Design review of the part built by this model. Coordinates are the model's own, in mm. Face numbers are marked on the shaded views. Round coordinates to 2 decimals unless told otherwise and drop trailing zeros. Use one line per item in the form item = value.
```python
from build123d import *

# Parameters (mm, degrees)
F0_W     = 539.75
F0_H     = 304.8
F0_W_2   = 15.24
F0_H_2   = 58.42
F0_W_3   = 304.8
F0_H_3   = 12.7
F0_R     = 47.625
F0_W_4   = 69.85
F0_H_4   = 7.62
F1_DEPTH = 12.7
F0_W_5   = 10.4902
F0_H_5   = 4.572
F2_DEPTH = 2.54
F0_R_2   = 41.275
F3_DEPTH = 12.7
F4_DEPTH = 5.08
F5_R     = 12.7
F6_R     = 5.08
F7_R     = 2.54
F8_R     = 2.032


with BuildPart() as f1:
    # F0 (on Top) → F1 (new body)
    with BuildSketch(Plane.XY):
        Rectangle(F0_W, F0_H)
        with Locations((-245.098478, -86.36)):
            Rectangle(F0_W_2, F0_H_2, mode=Mode.SUBTRACT)
        with Locations((-66.675, -107.95)):
            Rectangle(F0_W_3, F0_H_3, mode=Mode.SUBTRACT)
        with Locations((-66.675, -70.889322)):
            Rectangle(F0_W_3, F0_H_3, mode=Mode.SUBTRACT)
        with Locations((-66.675, -33.828645)):
            Rectangle(F0_W_3, F0_H_3, mode=Mode.SUBTRACT)
        with Locations((245.098478, -86.36)):
            Rectangle(F0_W_2, F0_H_2, mode=Mode.SUBTRACT)
        with Locations((-66.675, 3.232033)):
            Rectangle(F0_W_3, F0_H_3, mode=Mode.SUBTRACT)
        with Locations((-66.675, 40.292711)):
            Rectangle(F0_W_3, F0_H_3, mode=Mode.SUBTRACT)
        with Locations((-245.098478, 86.36)):
            Rectangle(F0_W_2, F0_H_2, mode=Mode.SUBTRACT)
        with Locations((-66.675, 77.353389)):
            Rectangle(F0_W_3, F0_H_3, mode=Mode.SUBTRACT)
        with Locations((-66.675, 114.414066)):
            Rectangle(F0_W_3, F0_H_3, mode=Mode.SUBTRACT)
        with Locations((177.8, 18.529066)):
            Circle(F0_R, mode=Mode.SUBTRACT)
        with Locations((245.098478, 86.36)):
            Rectangle(F0_W_2, F0_H_2, mode=Mode.SUBTRACT)
        with Locations((177.8, 120.764066)):
            Rectangle(F0_W_4, F0_H_4, mode=Mode.SUBTRACT)
    extrude(amount=F1_DEPTH)

    # F0 (on Top) → F2 (join)
    with BuildSketch(Plane.XY):
        with Locations((177.8, 120.764066)):
            Rectangle(F0_W_4, F0_H_4)
        with Locations((177.8, 120.764066)):
            Rectangle(F0_W_5, F0_H_5, mode=Mode.SUBTRACT)
    extrude(amount=F2_DEPTH)

    # F0 (on Top) → F3 (join)
    with BuildSketch(Plane.XY):
        with Locations((177.8, 18.529066)):
            Circle(F0_R)
        with Locations((177.8, 18.529066)):
            Circle(F0_R_2, mode=Mode.SUBTRACT)
    extrude(amount=F3_DEPTH)

    # F0 (on Top) → F4 (join)
    with BuildSketch(Plane.XY):
        with Locations((177.8, 18.529066)):
            Circle(F0_R_2)
    extrude(amount=F4_DEPTH)

    # F5
    f5_edges = [f1.edges().sort_by_distance(p)[0] for p in [
        (-269.875, 152.4, 6.35),
        (269.875, 152.4, 6.35),
        (269.875, -152.4, 6.35),
        (-269.875, -152.4, 6.35),
    ]]
    fillet(f5_edges, radius=F5_R)

    # F6
    f6_edges = [f1.edges().sort_by_distance(p)[0] for p in [
        (-219.075, 120.764066, 6.35),
        (85.725, 120.764066, 6.35),
        (-219.075, 33.942711, 6.35),
        (-219.075, -3.117967, 6.35),
        (-219.075, -40.178645, 6.35),
        (-219.075, -77.239322, 6.35),
        (-219.075, -114.3, 6.35),
        (-219.075, 108.064066, 6.35),
        (-219.075, 71.003389, 6.35),
        (85.725, 108.064066, 6.35),
        (85.725, 71.003389, 6.35),
        (85.725, 33.942711, 6.35),
        (85.725, -3.117967, 6.35),
        (85.725, -40.178645, 6.35),
        (85.725, -77.239322, 6.35),
        (85.725, -114.3, 6.35),
        (85.725, -101.6, 6.35),
        (85.725, -64.539322, 6.35),
        (85.725, -27.478645, 6.35),
        (85.725, 9.582033, 6.35),
        (85.725, 46.642711, 6.35),
        (85.725, 83.703389, 6.35),
        (-219.075, -101.6, 6.35),
        (-219.075, -64.539322, 6.35),
        (-219.075, -27.478645, 6.35),
        (-219.075, 9.582033, 6.35),
        (-219.075, 46.642711, 6.35),
        (-219.075, 83.703389, 6.35),
    ]]
    fillet(f6_edges, radius=F6_R)

    # F7
    f7_edges = [f1.edges().sort_by_distance(p)[0] for p in [
        (142.875, 124.574066, 7.62),
        (212.725, 124.574066, 7.62),
        (142.875, 116.954066, 7.62),
        (212.725, 116.954066, 7.62),
    ]]
    fillet(f7_edges, radius=F7_R)

    # F8
    f8_edges = [f1.edges().sort_by_distance(p)[0] for p in [
        (172.5549, 123.050066, 1.27),
        (183.0451, 123.050066, 1.27),
        (183.0451, 118.478066, 1.27),
        (172.5549, 118.478066, 1.27),
    ]]
    fillet(f8_edges, radius=F8_R)


solid = f1.part
```
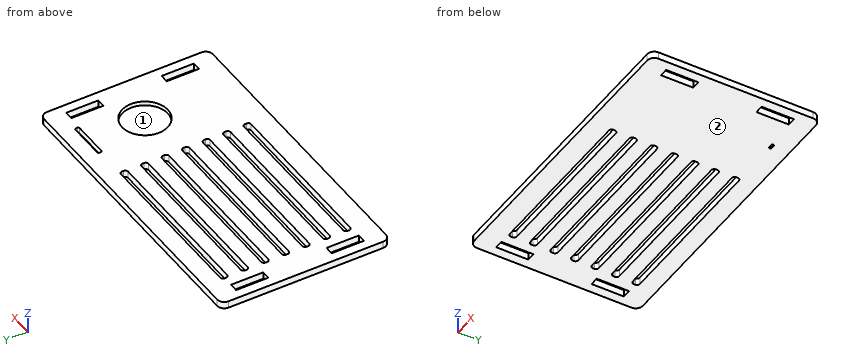
Q1. We need section A-A on x = 56.5. State how many separate pieces and enclosed holes the cut face has, then the cut area to 3 significant figures.
Calculated:
separate_pieces = 8
enclosed_holes = 0
area = 2,740 mm2
Q2. To check wall thickness, follow line 1 along Y through (x, z) = (177.8, 10.5); line 2 along X through (y, z) = (-84.5, 12) (3 decimals); line 3 along X through (y, z) = (-65, 0.75) (3 decimals). State the ranges of each line that lie inside material, in increasing order. Write a range as from..to.
Calculated:
line_1 = -152.4..-22.75, 59.8..116.95, 124.57..152.4
line_2 = -269.875..-252.718, -237.478..237.478, 252.718..269.875
line_3 = -269.875..-252.718, -237.478..-216.109, 82.759..237.478, 252.718..269.875
Q3. Draft analysis for pull direction X (two halves, no side actions). For the marked faces 1 and 2, state which applies: released by +X, released by -X, zero draft, split by the parting line, or undercut.
Calculated:
face_1 = undercut
face_2 = zero draft
